```python
from build123d import *

# Parameters (mm, degrees)
SKETCH1_W           = 349.25
SKETCH1_H           = 171.45
BOSS_EXTRUDE1_DEPTH = 85.725
CUT_EXTRUDE1_DEPTH  = 73.025
CUT_EXTRUDE2_REACH  = 87.725
SKETCH5_R           = 17.749738032
CUT_EXTRUDE3_REACH  = 351.25
SKETCH6_R           = 17.749738032
CHAMFER1_SIZE       = 0.635


with BuildPart() as part:
    # Sketch1 → Boss-Extrude1 (new body)
    with BuildSketch(Plane(origin=(0, 0, 0), x_dir=(1, 0, 0), z_dir=(0, 1, 0))):
        Rectangle(SKETCH1_W, SKETCH1_H)
    extrude(amount=BOSS_EXTRUDE1_DEPTH)

    # Sketch2 → Cut-Extrude1 (cut)
    with BuildSketch(Plane.XZ):
        with BuildLine():
            Line((143.166535328, 77.827138829), (-143.166535328, 77.827138829))
            ThreePointArc((-143.166535328, 77.827138829), (-159.826397833, 70.926397833), (-166.727138829, 54.266535328))
            Line((-166.727138829, 54.266535328), (-166.727138829, -54.266535328))
            ThreePointArc((-166.727138829, -54.266535328), (-159.826397833, -70.926397833), (-143.166535328, -77.827138829))
            Line((-143.166535328, -77.827138829), (143.166535328, -77.827138829))
            ThreePointArc((143.166535328, -77.827138829), (159.826397833, -70.926397833), (166.727138829, -54.266535328))
            Line((166.727138829, -54.266535328), (166.727138829, 54.266535328))
            ThreePointArc((166.727138829, 54.266535328), (159.826397833, 70.926397833), (143.166535328, 77.827138829))
        make_face()
    extrude(amount=-CUT_EXTRUDE1_DEPTH, mode=Mode.SUBTRACT)

    # Sketch5 → Cut-Extrude2 (cut, up to next)
    with BuildSketch(Plane(origin=(0, 85.725, 0), x_dir=(1, 0, 0), z_dir=(0, 1, 0)), mode=Mode.PRIVATE) as cut_extrude2_sk1:
        with Locations((13.724333657, 5.811180929)):
            Circle(SKETCH5_R)
    cut_extrude2_tool1 = extrude(cut_extrude2_sk1.sketch, amount=-CUT_EXTRUDE2_REACH, mode=Mode.PRIVATE) & part.part
    add(cut_extrude2_tool1.solids().sort_by_distance((13.724334, 85.725, -5.811181))[0], mode=Mode.SUBTRACT)

    # Sketch6 → Cut-Extrude3 (cut, up to next)
    with BuildSketch(Plane(origin=(174.625, 0, 0), x_dir=(0, 0, -1), z_dir=(1, 0, 0)), mode=Mode.PRIVATE) as cut_extrude3_sk1:
        with Locations((-1.47611621, 51.972642264)):
            Circle(SKETCH6_R)
    cut_extrude3_tool1 = extrude(cut_extrude3_sk1.sketch, amount=-CUT_EXTRUDE3_REACH, mode=Mode.PRIVATE) & part.part
    add(cut_extrude3_tool1.solids().sort_by_distance((174.625, 51.972642, 1.476116))[0], mode=Mode.SUBTRACT)

    # Chamfer1
    chamfer1_edges = [part.edges().sort_by_distance(p)[0] for p in [
        (159.826397833, 0, 70.926397833),
        (159.826397833, 0, -70.926397833),
        (-159.826397833, 0, -70.926397833),
        (0, 0, 77.827138829),
        (-159.826397833, 0, 70.926397833),
        (-166.727138829, 0, 0),
        (0, 0, -77.827138829),
        (166.727138829, 0, 0),
    ]]
    chamfer(chamfer1_edges, length=CHAMFER1_SIZE)


solid = part.part
```
Here's how the part is built. I have some questions about the finished solid (model axes, mm). A direction names the side the tool comes from. Round coordinates to 2 decimals unless told otherwise and drop trailing zeros. Order: outer loops, then holes, each group sorted by start corner. A loop starts at its lowest first (then second) coordinate and runs counter-clockwise, first axis right, second up. Notation, with made-up numbers: (-32, 36) -> (-2, 36) arc R18 cw to (-2, 47) -> close; hole circle Ø4 at (-12.5, 54). An arc over 180 degrees is marked (long way). Use a Markdown table: item, result. Add a question column.
(1) For pin 1 Ø21.5 at (y, z) = (51.97, 1.48) entering from +X; pin 2 Ø1 at (x, z) = (-41.5, 52.5) entering from -Y (3 decimals), each with a flat end and sliding along its axis, tell me the tip position at first contact or that it passes through.
(2) I need wall thicknesses on line 1 along X through (y, z) = (5, 43) (3 decimals); line 2 along Z through (x, y) = (-130.5, 61.5) (3 decimals); line 3 along X through (y, z) = (17.5, -72) (3 decimals). Which ranges of each line are inside material? Lowest first, please.
(3) For faces 1 (the face through (170.731, 34.645, 5.324)), 2 (the face through (30.654, 79.464, -11.143)), 3 (the face through (-160.01, 36.32, -70.74)), which set-ups out of +Z, -Z, +X, -X, +Y, -Y let a thin tool reach every point of the face, with its end or its side?
(4) If we mould it in two halves opening along Z, with no side actions, what happens to faces 4 (the face through (-2, 42, 85.725)), 5 (the face through (174.625, 33, 1)), 6 (the face through (159.64, 36.32, -71.11))? For each: released by +Z, released by -Z, zero draft, split by the parting line, or undercut.
(5) Suppose I cut it at C-C, the plane z = 39.5. Please give me the cut outline in (x, y) (3 decimals), and give its area (3 significant figures).
(6) Suppose I cut it at B-B, the plane x = 59. Please give me the cut outline in (y, z) (3 decimals).
(7) Suppose I cut it at A-A, the plane y = 30. Please give me the cut outline in (x, z) (3 decimals).
Verdict:
| question | item | result |
|---|---|---|
| 1 | pin 1 | x = -166.73 |
| 1 | pin 2 | y = 73.025 |
| 2 | line 1 | -174.625 to -166.727, 166.727 to 174.625 |
| 2 | line 2 | -85.725 to -77.827, 77.827 to 85.725 |
| 2 | line 3 | -174.625 to -158.679, 158.679 to 174.625 |
| 3 | face 1 | +X |
| 3 | face 2 | +Y, -Y |
| 3 | face 3 | -Y |
| 4 | face 4 | released by +Z |
| 4 | face 5 | zero draft |
| 4 | face 6 | undercut |
| 5 | outline | (-174.625, 0) -> (-167.362, 0) -> (-166.727, 0.635) -> (-166.727, 73.025) -> (166.727, 73.025) -> (166.727, 0.635) -> (167.362, 0) -> (174.625, 0) -> (174.625, 85.725) -> (-174.625, 85.725) -> close |
| 5 | area | 5,590 mm2 |
| 6 | outline | (0, -85.725) -> (85.725, -85.725) -> (85.725, 85.725) -> (0, 85.725) -> (0, 78.462) -> (0.635, 77.827) -> (73.025, 77.827) -> (73.025, -77.827) -> (0.635, -77.827) -> (0, -78.462) -> close |
| 7 | outline | (-174.625, -85.725) -> (174.625, -85.725) -> (174.625, 85.725) -> (-174.625, 85.725) -> close; hole (-166.727, -54.267) arc R23.561 ccw to (-143.167, -77.827) -> (143.167, -77.827) arc R23.561 ccw to (166.727, -54.267) -> (166.727, 54.267) arc R23.561 ccw to (143.167, 77.827) -> (-143.167, 77.827) arc R23.561 ccw to (-166.727, 54.267) -> close |
